Work out the finished part from the listing and answer in its coordinate system (mm). A direction names the side the tool comes from. Round coordinates to 2 decimals unless told otherwise and drop trailing zeros. Order: outer loops, then holes, each group sorted by start corner. A loop starts at its lowest first (then second) coordinate and runs counter-clockwise, first axis right, second up. Notation, with made-up numbers: (-30.75, 7.25) - (-19.75, 7.25) arc R16 cw to (-19.75, 34.25) - close; hole circle Ø3 at (-20, -32.5). An arc over 180 degrees is marked (long way). Put each result on its own line as item: value.
```python
from build123d import *

# Parameters (mm, degrees)
SKETCH1_W             = 350
SKETCH1_H             = 300
BOSS_EXTRUDE1_DEPTH   = 100
SHELL1_T              = -3
SKETCH2_R             = 11
CUT_EXTRUDE1_DEPTH    = 10
SKETCH3_R             = 11
CUT_EXTRUDE2_DEPTH    = 10
SKETCH4_R             = 11
CUT_EXTRUDE3_DEPTH    = 10
FILLET1_R             = 40
FILLET2_R             = 5
SKETCH5_R             = 10
BOSS_EXTRUDE2_DEPTH   = 15
SKETCH6_R             = 17.5
BOSS_EXTRUDE3_DEPTH   = 15
CHAMFER1_SIZE         = 10
EXTRUDE_THIN1_DEPTH   = 10
EXTRUDE_THIN1_START   = 50
EXTRUDE_THIN1_2_DEPTH = 10
EXTRUDE_THIN1_START_2 = 10
EXTRUDE_THIN1_3_DEPTH = 40
SKETCH8_W             = 100
SKETCH8_H             = 60
CUT_EXTRUDE4_DEPTH    = 10
SKETCH9_R             = 6
CUT_EXTRUDE5_DEPTH    = 10


# Read off the part's stored shape, not the designer's step: Extrude-Thin1
with BuildPart() as part:
    # Sketch1 → Boss-Extrude1 (new body)
    with BuildSketch(Plane(origin=(0, 0, 0), x_dir=(1, 0, 0), z_dir=(0, 1, 0))):
        Rectangle(SKETCH1_W, SKETCH1_H)
    extrude(amount=BOSS_EXTRUDE1_DEPTH)

    # Shell1
    shell1_openings = [part.faces().sort_by_distance(p)[0] for p in [
        (0, 100, 0),
    ]]
    offset(amount=SHELL1_T, openings=shell1_openings, kind=Kind.INTERSECTION)

    # Sketch2 → Cut-Extrude1 (cut)
    with BuildSketch(Plane.ZY.offset(175)):
        with Locations((80, 23)):
            Circle(SKETCH2_R)
        with Locations((15, 23)):
            Circle(SKETCH2_R)
    extrude(amount=-CUT_EXTRUDE1_DEPTH, mode=Mode.SUBTRACT)

    # Sketch3 → Cut-Extrude2 (cut)
    with BuildSketch(Plane.XY.offset(150)):
        with Locations((43.31, 23)):
            Circle(SKETCH3_R)
    extrude(amount=-CUT_EXTRUDE2_DEPTH, mode=Mode.SUBTRACT)

    # Sketch4 → Cut-Extrude3 (cut)
    with BuildSketch(Plane(origin=(175, 0, 0), x_dir=(0, 0, -1), z_dir=(1, 0, 0))):
        with Locations((50, 23)):
            Circle(SKETCH4_R)
    extrude(amount=-CUT_EXTRUDE3_DEPTH, mode=Mode.SUBTRACT)

    # Fillet1
    fillet1_edges = [part.edges().sort_by_distance(p)[0] for p in [
        (172, 51.5, 147),
        (172, 51.5, -147),
        (-172, 51.5, -147),
        (-172, 51.5, 147),
        (175, 50, 150),
        (-175, 50, 150),
        (-175, 50, -150),
        (175, 50, -150),
    ]]
    fillet(fillet1_edges, radius=FILLET1_R)

    # Fillet2
    fillet2_edges = [part.edges().sort_by_distance(p)[0] for p in [
        (0, 0, -150),
        (175, 0, 0),
        (0, 0, 150),
        (-175, 0, 0),
        (-163.284271247, 0, 138.284271247),
        (163.284271247, 0, 138.284271247),
        (-163.284271247, 0, -138.284271247),
        (163.284271247, 0, -138.284271247),
    ]]
    fillet(fillet2_edges, radius=FILLET2_R)

    # Sketch5 → Boss-Extrude2 (add)
    with BuildSketch(Plane.XZ):
        with Locations(Location((-135, -110, 0), (0, 0, 90))):
            Circle(SKETCH5_R)
        with Locations(Location((-135, 110, 0), (0, 0, 90))):
            Circle(SKETCH5_R)
        with Locations(Location((135, -110, 0), (0, 0, 90))):
            Circle(SKETCH5_R)
        with Locations(Location((135, 110, 0), (0, 0, 90))):
            Circle(SKETCH5_R)
    extrude(amount=BOSS_EXTRUDE2_DEPTH)

    # Sketch6 → Boss-Extrude3 (add)
    with BuildSketch(Plane.XZ.offset(15)):
        with Locations(Location((135, 110, 0), (0, 0, 270))):
            Circle(SKETCH6_R)
        with Locations(Location((135, -110, 0), (0, 0, 270))):
            Circle(SKETCH6_R)
        with Locations(Location((-135, 110, 0), (0, 0, 270))):
            Circle(SKETCH6_R)
        with Locations(Location((-135, -110, 0), (0, 0, 270))):
            Circle(SKETCH6_R)
    extrude(amount=BOSS_EXTRUDE3_DEPTH)

    # Chamfer1
    # the kernel refuses this chamfer: 10 mm, written as the material it takes off along each edge
    with BuildSketch(Plane(origin=(-135, -15, -110), x_dir=(0, 0, -1), z_dir=(-1, 0, 0))) as chamfer1_piece_1_section:
        Polygon((17.5 - CHAMFER1_SIZE, 0), (17.5, CHAMFER1_SIZE), (17.5, 0), align=None)
    chamfer1_piece_1 = revolve(axis=Axis((-135, -15, -110), (0, -1, 0)), mode=Mode.PRIVATE)
    chamfer1_piece_1 = chamfer1_piece_1 - Plane(origin=(-135, -21.273186291, -110), x_dir=(0, 0, 1), z_dir=(0, 1, 0)) * Cylinder(10, 70, mode=Mode.PRIVATE)
    add(chamfer1_piece_1, mode=Mode.SUBTRACT)
    with BuildSketch(Plane(origin=(-135, -15, 110), x_dir=(0, 0, -1), z_dir=(-1, 0, 0))) as chamfer1_piece_2_section:
        Polygon((17.5 - CHAMFER1_SIZE, 0), (17.5, CHAMFER1_SIZE), (17.5, 0), align=None)
    chamfer1_piece_2 = revolve(axis=Axis((-135, -15, 110), (0, -1, 0)), mode=Mode.PRIVATE)
    chamfer1_piece_2 = chamfer1_piece_2 - Plane(origin=(-135, -21.273186291, 110), x_dir=(0, 0, 1), z_dir=(0, 1, 0)) * Cylinder(10, 70, mode=Mode.PRIVATE)
    add(chamfer1_piece_2, mode=Mode.SUBTRACT)
    with BuildSketch(Plane(origin=(135, -15, -110), x_dir=(0, 0, -1), z_dir=(-1, 0, 0))) as chamfer1_piece_3_section:
        Polygon((17.5 - CHAMFER1_SIZE, 0), (17.5, CHAMFER1_SIZE), (17.5, 0), align=None)
    chamfer1_piece_3 = revolve(axis=Axis((135, -15, -110), (0, -1, 0)), mode=Mode.PRIVATE)
    chamfer1_piece_3 = chamfer1_piece_3 - Plane(origin=(135, -21.273186291, -110), x_dir=(0, 0, 1), z_dir=(0, 1, 0)) * Cylinder(10, 71, mode=Mode.PRIVATE)
    add(chamfer1_piece_3, mode=Mode.SUBTRACT)
    with BuildSketch(Plane(origin=(135, -15, 110), x_dir=(0, 0, -1), z_dir=(-1, 0, 0))) as chamfer1_piece_4_section:
        Polygon((17.5, CHAMFER1_SIZE), (17.5 - CHAMFER1_SIZE, 0), (17.5, 0), align=None)
    chamfer1_piece_4 = revolve(axis=Axis((135, -15, 110), (0, -1, 0)), mode=Mode.PRIVATE)
    chamfer1_piece_4 = chamfer1_piece_4 - Plane(origin=(135, -21.273186291, 110), x_dir=(0, 0, 1), z_dir=(0, 1, 0)) * Cylinder(10, 71, mode=Mode.PRIVATE)
    add(chamfer1_piece_4, mode=Mode.SUBTRACT)

    # Extrude-Thin1 outline → Extrude-Thin1 (add)
    with BuildSketch(Plane(origin=(0, 3, 0), x_dir=(1, 0, 0), z_dir=(0, 1, 0))):
        with BuildLine():
            Line((-172, 27), (-2, 27))
            Line((-2, 27), (-2, 147))
            Line((-2, 147), (-132, 147))
            ThreePointArc((-132, 147), (-160.284271247, 135.284271247), (-172, 107))
            Line((-172, 107), (-172, 27))
        make_face()
    extrude(amount=EXTRUDE_THIN1_DEPTH)

    # Extrude-Thin1 2 outline → Extrude-Thin1 2 (add)
    with BuildSketch(Plane(origin=(0, 3, 0), x_dir=(1, 0, 0), z_dir=(0, 1, 0)).offset(EXTRUDE_THIN1_START)):
        with BuildLine():
            Line((-172, 27), (-2, 27))
            Line((-2, 27), (-2, 147))
            Line((-2, 147), (-132, 147))
            ThreePointArc((-132, 147), (-160.284271247, 135.284271247), (-172, 107))
            Line((-172, 107), (-172, 27))
        make_face()
    extrude(amount=EXTRUDE_THIN1_2_DEPTH)

    # Extrude-Thin1 3 outline → Extrude-Thin1 3 (add)
    with BuildSketch(Plane(origin=(0, 3, 0), x_dir=(1, 0, 0), z_dir=(0, 1, 0)).offset(EXTRUDE_THIN1_START_2)):
        with BuildLine():
            Line((-172, 27), (-2, 27))
            Line((-2, 27), (-2, 147))
            Line((-2, 147), (-132, 147))
            ThreePointArc((-132, 147), (-160.284271247, 135.284271247), (-172, 107))
            Line((-172, 107), (-172, 27))
        make_face()
        with BuildLine():
            ThreePointArc((-169, 107), (-158.162950904, 133.162950904), (-132, 144))
            Line((-132, 144), (-5, 144))
            Line((-5, 144), (-5, 30))
            Line((-5, 30), (-169, 30))
            Line((-169, 30), (-169, 107))
        make_face(mode=Mode.SUBTRACT)
    extrude(amount=EXTRUDE_THIN1_3_DEPTH)

    # Sketch8 → Cut-Extrude4 (cut)
    with BuildSketch(Plane.ZY.offset(175)):
        with Locations((-60, 55)):
            Rectangle(SKETCH8_W, SKETCH8_H)
    extrude(amount=-CUT_EXTRUDE4_DEPTH, mode=Mode.SUBTRACT)

    # Sketch9 → Cut-Extrude5 (cut)
    with BuildSketch(Plane.XY.offset(150)):
        with Locations((-105, 55)):
            Circle(SKETCH9_R)
        with Locations((-25, 55)):
            Circle(SKETCH9_R)
    extrude(amount=-CUT_EXTRUDE5_DEPTH, mode=Mode.SUBTRACT)


solid = part.part
```
1) A cutting plane is placed at C-C on y = 38. Write down the section's boundary in (x, z), then the cut area to 3 significant figures.
Findings below:
outline: (-175, -110) arc R40 ccw to (-135, -150) - (135, -150) arc R40 ccw to (175, -110) - (175, 110) arc R40 ccw to (135, 150) - (-135, 150) arc R40 ccw to (-175, 110) - (-175, -10) - (-172, -10) - (-172, 107) arc R40 cw to (-132, 147) - (132, 147) arc R40 cw to (172, 107) - (172, -107) arc R40 cw to (132, -147) - (-2, -147) - (-2, -27) - (-165, -27) - (-165, -30) - (-5, -30) - (-5, -144) - (-132, -144) arc R37 cw to (-168.88, -110) - close
area: 4,960 mm2
2) Straight lines are drawn through the part: L1, parallel to Z at x = -43, y = 49.5; L2, parallel to Y at x = -93, z = -59; L3, parallel to X at y = 90, z = -97. For each, find the intervals that lie inside material, in ascending order. Write a range as from..to.
Findings below:
L1: z = -150..-144, -30..-27, 147..150
L2: y = 0..13, 53..63
L3: x = -175..-172, 172..175
3) For a pull along X with two mould halves and no side action, classify faces 1 (the cylindrical face through (162.972, 53.165, 138.594)), 2 (the conical face through (-144.29, -17.97, -114.83)), 3 (the cylindrical face through (173.521, 13.241, -55.076)) as pulls with the +X half, pulls with the -X half, needs draft (parallel to the pull), parting line crosses it, or undercut.
Findings below:
face 1: pulls with the +X half
face 2: undercut
face 3: needs draft
4) A cutting plane is placed at A-A on x = -25. Write down the section's boundary in (y, z).
Findings below:
outline: (0, -145) arc R5 ccw to (5, -150) - (100, -150) - (100, -147) - (63, -147) - (63, -27) - (3, -27) - (3, 147) - (49, 147) - (49, 150) - (5, 150) arc R5 ccw to (0, 145) - close; (61, 147) - (100, 147) - (100, 150) - (61, 150) - close; hole (13, -144) - (53, -144) - (53, -30) - (13, -30) - close
5) Given pin 1 Ø20 at (y, z) = (23, 15) entering from -X; pin 2 Ø8 at (x, z) = (-135, -35) entering from -Y; pin 3 Ø9.5 at (y, z) = (19.5, -52.5) entering from +X, each flat-ended and moving along its own axis, determine where each tip first touches the part or whether it passes through.
Findings below:
pin 1: stops at x = 172
pin 2: stops at y = 0
pin 3: stops at x = -2
6) A cutting plane is placed at D-D on y = -10. Write down the section's boundary in (x, z), then the cut area to 3 significant figures.
Findings below:
outline: circle Ø20 at (-135, -110); circle Ø20 at (-135, 110); circle Ø20 at (135, -110); circle Ø20 at (135, 110)
area: 1,260 mm2
7) A cutting plane is placed at B-B on z = 80. Write down the section's boundary in (x, y), then the cut area to 3 significant figures.
Findings below:
outline: (-175, 5) arc R5 ccw to (-170, 0) - (170, 0) arc R5 ccw to (175, 5) - (175, 100) - (172, 100) - (172, 3) - (-172, 3) - (-172, 12) - (-175, 12) - close; (-175, 34) - (-172, 34) - (-172, 100) - (-175, 100) - close
area: 1,560 mm2
8) For faces 4 (the flat face through (-165, 54, -66)), 5 (the flat face through (27, 62, -147)), 6 (the cylindrical face through (-120.244, -27.465, 100.592)), 7 (the conical face through (125.71, -17.97, -114.83)), 8 (the flat face through (-172, 25, -61)), determine the directions among +Z, -Z, +X, -X, +Y, -Y from which every point of the face is accessible in a straight line to the end or side of a thin tool.
Findings below:
face 4: -X, +Y
face 5: +Y
face 6: -Y
face 7: none
face 8: -X
